Read the model definition and answer for the solid it produces. Units are mm, in the model's axes. A direction names the side the tool comes from. Give positions to 0.01 mm unless a question says otherwise; leave off trailing zeros. Write each loop counter-clockwise with the first axis right and the second up, starting at its lowest first coordinate (ties: lowest second). Pieces come first, ordered by that corner, then holes.
Autodesk Inventor part; units mm, degrees
ref_plane "YZ Plane" through (0, 0, 0) normal (1, 0, 0) x (0, 1, 0)
ref_plane "XZ Plane" through (0, 0, 0) normal (0, 1, 0) x (-1, 0, 0)
ref_plane "XY Plane" through (0, 0, 0) normal (0, 0, 1) x (1, 0, 0)
sketch "Náčrt1" plane through (0, 0, 0) normal (0, 0, 1) x (1, 0, 0)
  circle A0 centre (0, 0) radius 5.25
  circle A1 centre (0, 0) radius 8.25
  line L0 (5.25, 0) -> (8.25, 0)
  line L1 (-8.25, 0) -> (-48.25, 0)
  line L2 (-8.25, 0) -> (-5.25, 0)
  line L3 (-48.25, 0) -> (-48.25, 2)
  line L4 (-48.25, 2) -> (-8.0039, 2)
  dimension "d0" = 10.5
  dimension "d1" = 3
  dimension "d2" = 40
  dimension "d3" = 2
extrude "Vysunutí1" add sketch "Náčrt1" along normal blind 65 contours A0 L2 A1 L0 | L1 L3 L4 A1 picked at (7.1703, 0.6574)
sketch "Náčrt2" plane through (-48.25, 2, 0) normal (0, 1, 0) x (1, 0, 0)
  line L0 (40.2461, 0) -> (40.2461, -65)
  line L1 (56.5, 0) -> (56.5, -65)
  line L2 (40.2461, -10) -> (56.5, -10)
  line L3 (56.5, -10) -> (56.5, -55)
  line L4 (56.5, -55) -> (40.2461, -55)
  line L5 (40.2461, -55) -> (40.2461, -10)
  line L6 (40.2461, 0) -> (56.5, 0)
  line L7 (40.2461, -65) -> (56.5, -65)
  point P0 (48.25, 0)
  dimension "d6" = 10
  dimension "d7" = 10
extrude "Vysunutí2" cut sketch "Náčrt2" along normal mid plane 65 contours L2 L1 L4 L0
sketch "Náčrt3" plane through (-48.25, 2, 0) normal (0, 1, 0) x (1, 0, 0)
  line L0 (0, 0) -> (0, -65)
  line L1 (40.2461, 0) -> (0, 0)
  line L2 (0, 0) -> (40.2461, 0)
  line L3 (40.2461, -65) -> (56.5, -65)
  line L4 (40.2461, 0) -> (40.2461, -65)
  line L5 (40.2461, -65) -> (38.2461, -65)
  line L6 (38.2461, -65) -> (38.2461, -2)
  line L7 (38.2461, -2) -> (2, -2)
  line L8 (2, -2) -> (2, -65)
  line L9 (0, -65) -> (2, -65)
  line L10 (0, -65) -> (0, 0)
  point P0 (48.25, 0)
  dimension "d10" = 2
  dimension "d11" = 2
  dimension "d12" = 2
  dimension "d13" = 2
  dimension "d14" = 2
extrude "Vysunutí3" add sketch "Náčrt3" along normal blind 8
fillet "Zaoblení1" radius 2 2 edges at (-10.0039, 6, 2) (-46.25, 6, 2)
fillet "Zaoblení2" radius 1 2 edges at (-48.25, 5, 65) (-48.25, 5, 0)
fillet "Zaoblení3" radius 1 2 edges at (-46.25, 6, 65) (-10.0039, 6, 65)
properties part number "DripCatcher"
Item 1: Each of these flat-tipped pins is pushed along its axis until it touches: pin 1 Ø2.5 at (x, y) = (-35.5, 4.5) entering from +Z; pin 2 Ø4 at (y, z) = (7.5, 40) entering from +X. Where does it stop, or does it pass through?
Result set:
pin 1: stops at z = 2
pin 2: stops at x = -8
Item 2: Section C-C (z = 24.5) is taken. Write down the section's boundary in (x, y).
Result set:
outline: (-48.25, 0) - (-8, 0) - (-8, 10) - (-10, 10) - (-10, 2) - (-46.25, 2) - (-46.25, 10) - (-48.25, 10) - close
Item 3: Determine the mould class of faces 1 (the flat face through (-48.25, 5, 32)), 2 (the flat face through (7, 0, 60)), 3 (the cylindrical face through (-0.12, 5.25, 59.93)) for opening direction X: pulls with the +X half, pulls with the -X half, needs draft (parallel to the pull), parting line crosses it, or undercut.
Result set:
face 1: pulls with the -X half
face 2: needs draft
face 3: undercut
Item 4: Find the intervals of material crossed by line 1 along X through (y, z) = (6.75, 51.5); line 2 along X through (y, z) = (7.5, 4.5); line 3 along Z through (x, y) = (-20.5, 8.25), in increasing order.
Result set:
line 1: x = -48.25 to -46.25, -10 to -8
line 2: x = -48.25 to -46.25, -10 to -8, -3.44 to 3.44
line 3: z = 0 to 2
Item 5: Section A-A (x = 0) is taken. Write down the section's boundary in (y, z).
Result set:
outline: (5.25, 0) - (8.25, 0) - (8.25, 10) - (5.25, 10) - close; (5.25, 55) - (8.25, 55) - (8.25, 65) - (5.25, 65) - close
Item 6: Section D-D (x = -40.5) is taken. Write down the section's boundary in (y, z), and give its area (3 significant figures).
Result set:
outline: (0, 0) - (10, 0) - (10, 2) - (2, 2) - (2, 65) - (0, 65) - close
area: 146 mm2
Item 7: Which of the six approach directions +Z, -Z, +X, -X, +Y, -Y give full straight-line access (tool end or side, diameter ignored) to faces 4 (the flat face through (0, 6, 10)), 5 (the flat face through (-28, 2, 33)), 6 (the flat face through (-48, 10, 23))?
Result set:
face 4: +X, +Y, -Y
face 5: +Z, +Y
face 6: +Z, -Z, +X, -X, +Y
